Input: dimensioned drawing with shaded views. Units: mm. Origin: part minimum x, y, z. A direction names the side the tool comes from. Coordinates: 2 decimals unless noted, no trailing zeros. Loops run counter-clockwise (first coordinate to the right, second up) from the corner with the lowest first, then second, coordinate; pieces in that order, holes last.
Item 1: Contact query for flat-ended pins moving along their axis: P1, Ø3, axis at y = 6.5, z = 6.5, coming from the -X side; P2, Ø6, axis at x = 23, y = 6, coming from the -Z side; P3, Ø5, axis at y = 9, z = 10, coming from the +X side; P4, Ø5, axis at x = 20, y = 10, coming from the +Z side. Output: stop coordinate, or through.
Item 2: Section C-C on x = 36. Return loops of the section in (y, z).
Item 3: Section D-D on z = 7.75. Return loops of the section in (x, y).
Item 4: Ray query, line 1 along Y through (x, z) = (36, 1.5); line 2 along Y through (x, z) = (27, 8.5); line 3 along X through (y, z) = (12.25, 5.75). Return the intervals inside material, ascending.
Item 5: Section A-A on y = 10. Return loops of the section in (x, z).
Item 6: Section B-B on z = 2.75. Return loops of the section in (x, y).
Item 7: Pull-direction query (X, two-part tool) for the marked faces 6, 7, 8 and 9; classes: released by +X, released by -X, zero draft, split by the parting line, or undercut.
Item 8: Reachability of the marked faces 1, 2, 3, 4 and 5 from +Z, -Z, +X, -X, +Y, -Y: full face, straight path, thin tool, end or side. Return the list, or none.
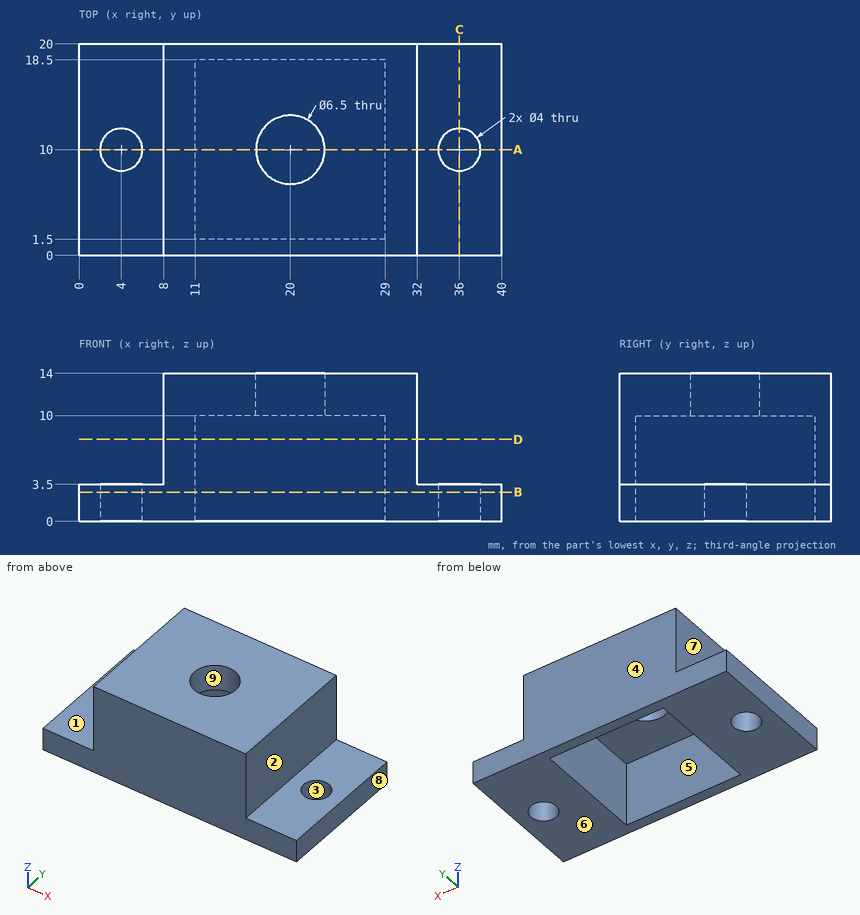
Results found:
1. P1: stops at x = 8
1. P2: stops at z = 10
1. P3: stops at x = 32
1. P4: passes through
2. outline: (0, 0) - (8, 0) - (8, 3.5) - (0, 3.5) - close; (12, 0) - (20, 0) - (20, 3.5) - (12, 3.5) - close
3. outline: (8, 0) - (32, 0) - (32, 20) - (8, 20) - close; hole (11, 1.5) - (29, 1.5) - (29, 18.5) - (11, 18.5) - close
4. line 1: y = 0 to 8, 12 to 20
4. line 2: y = 0 to 1.5, 18.5 to 20
4. line 3: x = 8 to 11, 29 to 32
5. outline: (0, 0) - (2, 0) - (2, 3.5) - (0, 3.5) - close; (6, 0) - (11, 0) - (11, 10) - (16.75, 10) - (16.75, 14) - (8, 14) - (8, 3.5) - (6, 3.5) - close; (23.25, 10) - (29, 10) - (29, 0) - (34, 0) - (34, 3.5) - (32, 3.5) - (32, 14) - (23.25, 14) - close; (38, 0) - (40, 0) - (40, 3.5) - (38, 3.5) - close
6. outline: (0, 0) - (40, 0) - (40, 20) - (0, 20) - close; hole circle Ø4 at (4, 10); hole (11, 1.5) - (29, 1.5) - (29, 18.5) - (11, 18.5) - close; hole circle Ø4 at (36, 10)
7. face 6: zero draft
7. face 7: released by -X
7. face 8: released by +X
7. face 9: undercut
8. face 1: +Z, -X, +Y, -Y
8. face 2: +Z, +X, +Y, -Y
8. face 3: +Z, -Z
8. face 4: +Z, -Z, +X, -X, +Y
8. face 5: -Z
